Part print with two shaded views. Sizes in mm from the minimum x, y, z corner. A direction names the side the tool comes from. Round coordinates to 2 decimals unless told otherwise and drop trailing zeros. Order: outer loops, then holes, each group sorted by start corner. A loop starts at its lowest first (then second) coordinate and runs counter-clockwise, first axis right, second up. Notation, with made-up numbers: (22, -39) -> (81, -39) arc R21 ccw to (81, -24) -> close; hole circle Ø3 at (45.25, -27.75). An arc over 180 degrees is marked (long way). Answer as a JSON object with one key per item and string values.
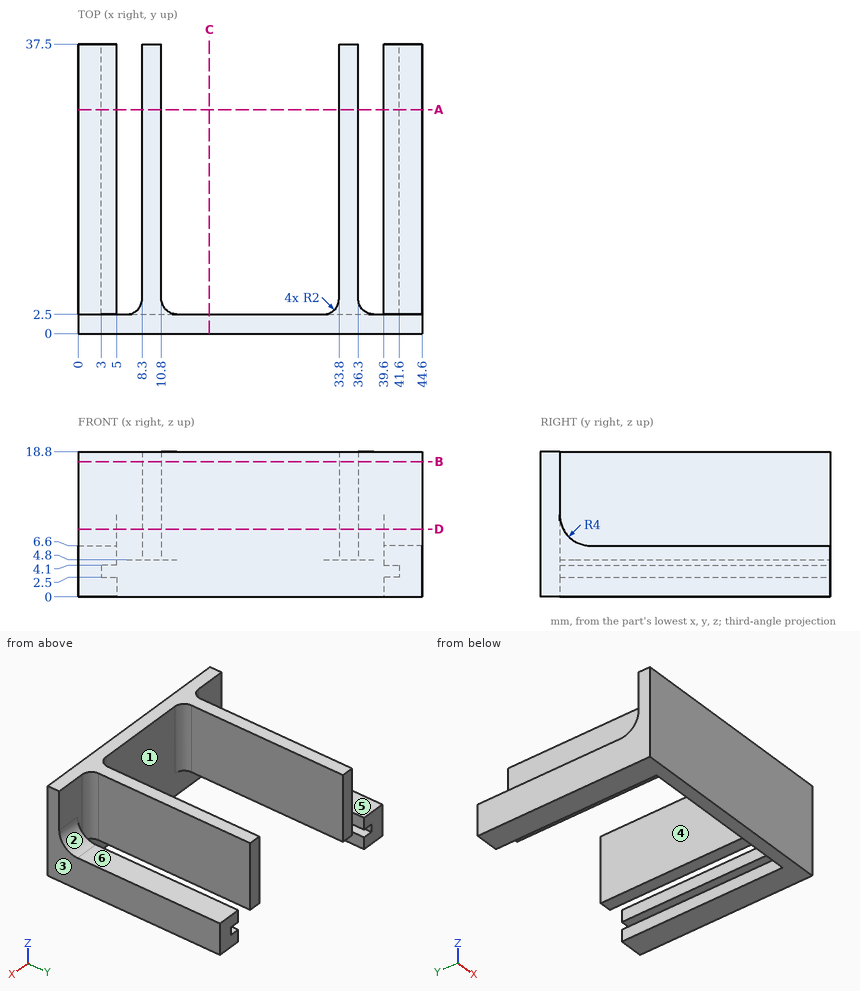
1) Cut at A-A, the plane y = 29. Give the cut face in (x, z).
Checked values:
{"outline": "(0, 0) -> (5, 0) -> (5, 2.5) -> (3, 2.5) -> (3, 4.1) -> (5, 4.1) -> (5, 6.6) -> (0, 6.6) -> close; (8.3, 4.8) -> (10.8, 4.8) -> (10.8, 18.8) -> (8.3, 18.8) -> close; (33.8, 4.8) -> (36.3, 4.8) -> (36.3, 18.8) -> (33.8, 18.8) -> close; (39.6, 0) -> (44.6, 0) -> (44.6, 6.6) -> (39.6, 6.6) -> (39.6, 4.1) -> (41.6, 4.1) -> (41.6, 2.5) -> (39.6, 2.5) -> close"}
2) Cut at D-D, the plane z = 8.75. Give the cut face in (x, y), plus the area to 3 significant figures.
Checked values:
{"outline": "(0, 0) -> (44.6, 0) -> (44.6, 2.95) -> (39.6, 2.95) -> (39.6, 2.5) -> (38.3, 2.5) arc R2 cw to (36.3, 4.5) -> (36.3, 37.5) -> (33.8, 37.5) -> (33.8, 4.5) arc R2 cw to (31.8, 2.5) -> (12.8, 2.5) arc R2 cw to (10.8, 4.5) -> (10.8, 37.5) -> (8.3, 37.5) -> (8.3, 4.5) arc R2 cw to (6.3, 2.5) -> (5, 2.5) -> (5, 2.95) -> (0, 2.95) -> close", "area": "294 mm²"}
3) Flat gauge pins, fed straight in: pin 1 Ø3 at (x, z) = (6.5, 11.5) entering from +Y; pin 2 Ø4 at (y, z) = (26.5, 12) entering from -X; pin 3 Ø5 at (y, z) = (5.5, 12) entering from +X. Where does each tip first touch, or does it go through?
Checked values:
{"pin 1": "stops at y = 3.45", "pin 2": "stops at x = 8.3", "pin 3": "stops at x = 36.98"}
4) Pull direction X, two halves, no side cores. Call the marked faces 1, 2 and 3: pulls with the +X half, pulls with the -X half, needs draft (parallel to the pull), parting line crosses it, or undercut.
Checked values:
{"face 1": "undercut", "face 2": "needs draft", "face 3": "pulls with the +X half"}
5) Cut at C-C, the plane x = 17. Give the cut face in (y, z), plus the area to 3 significant figures.
Checked values:
{"outline": "(0, 0) -> (2.5, 0) -> (2.5, 18.8) -> (0, 18.8) -> close", "area": "47.0 mm²"}
6) Probe L1, parallel to X at y = 17.5, z = 16.5; L2, parallel to Z at x = 41.5, y = 17.5; L3, parallel to Y at x = 15, z = 2. List the from-to ranges inside material, lowest first. Write a range as from..to.
Checked values:
{"L1": "x = 8.3..10.8, 33.8..36.3", "L2": "z = 0..2.5, 4.1..6.6", "L3": "y = 0..2.5"}
7) Cut at B-B, the plane z = 17.5. Give the cut face in (x, y), plus the area to 3 significant figures.
Checked values:
{"outline": "(0, 0) -> (44.6, 0) -> (44.6, 2.5) -> (38.3, 2.5) arc R2 cw to (36.3, 4.5) -> (36.3, 37.5) -> (33.8, 37.5) -> (33.8, 4.5) arc R2 cw to (31.8, 2.5) -> (12.8, 2.5) arc R2 cw to (10.8, 4.5) -> (10.8, 37.5) -> (8.3, 37.5) -> (8.3, 4.5) arc R2 cw to (6.3, 2.5) -> (0, 2.5) -> close", "area": "290 mm²"}
8) Which spindle directions (+Z, -Z, +X, -X, +Y, -Y) get a long thin tool onto all of the face, cutting with end or side? Do the marked faces 4, 5 and 6. Say none if no direction does.
Checked values:
{"face 4": "+Z, -Z, +Y", "face 5": "+Z, -X, +Y", "face 6": "+Z, +X, +Y"}
